Could you check a few things on this drawing? It's one solid part, dimensions in mm from its lowest x, y, z. Give positions to 0.01 mm unless a question says otherwise; leave off trailing zeros. Loops run counter-clockwise (first coordinate to the right, second up) from the corner with the lowest first, then second, coordinate; pieces in that order, holes last. Notation, with made-up numbers: M -20,35 L 5,35 A17 cw 5,43 Z; hole C -23,78.5 d5. An arc over 180 degrees is marked long. Answer in a Markdown table with one row per item. Add a question column.
1. I need wall thicknesses on line 1 along Z through (x, y) = (30, 6); line 2 along X through (y, z) = (14.25, 131); line 3 along Z through (x, y) = (31, 2.5). Which ranges of each line are inside material? Lowest first, please. Write a range as from..to.
2. If we section it at C-C on z = 130: List the corners of the cut face in (x, y) for me.
3. If we section it at B-B on y = 18.5: List the corners of the cut face in (x, z) for me, then the cut area to 3 significant figures.
4. I'm going to push a flat-ended pin straight in: pin 1 Ø12 at (x, z) = (45, 85.5) entering from -Y. Where does the tip first touch, or does it pass through?
5. If we section it at A-A on x = 30: List the corners of the cut face in (y, z) for me, then the cut area to 3 significant figures.
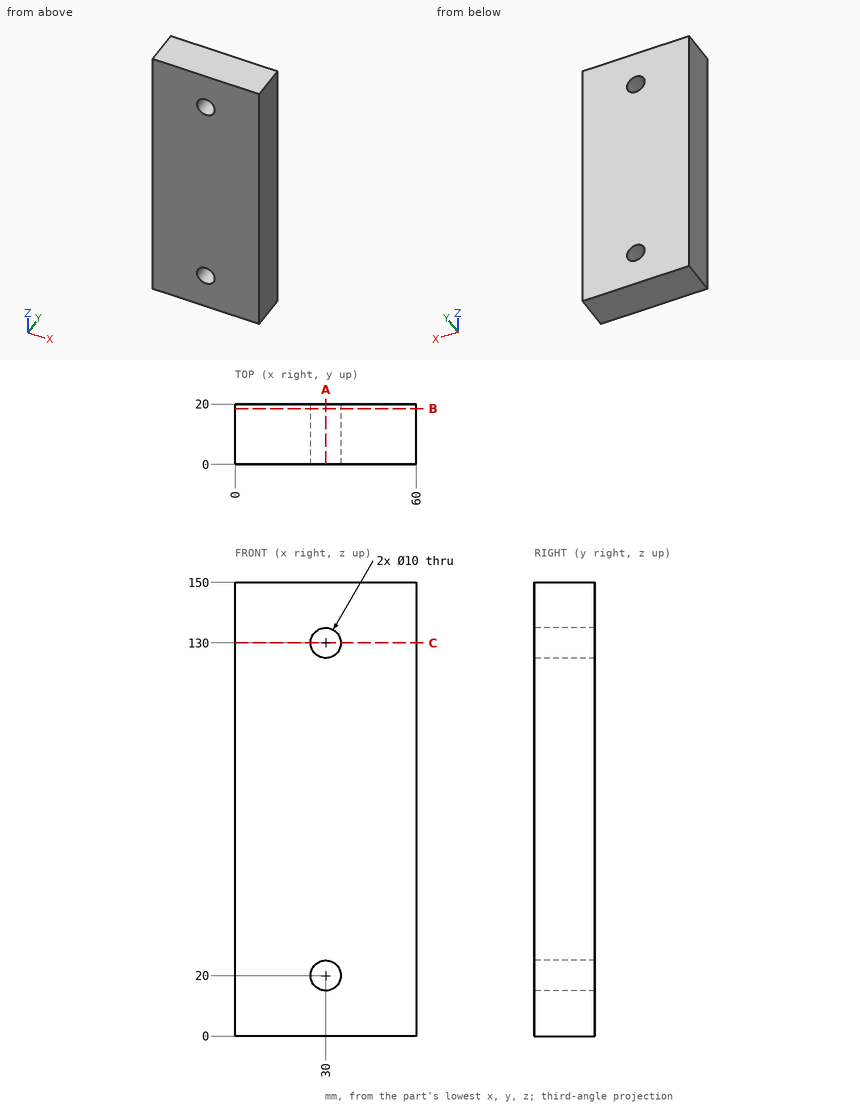
Results:
| question | item | result |
|---|---|---|
| 1 | line 1 | 0..15, 25..125, 135..150 |
| 1 | line 2 | 0..25.1, 34.9..60 |
| 1 | line 3 | 0..15.1, 24.9..125.1, 134.9..150 |
| 2 | outline | M 0,0 L 25,0 L 25,20 L 0,20 Z; M 35,0 L 60,0 L 60,20 L 35,20 Z |
| 3 | outline | M 0,0 L 60,0 L 60,150 L 0,150 Z; hole C 30,20 d10; hole C 30,130 d10 |
| 3 | area | 8,840 mm2 |
| 4 | pin 1 | y = 0 |
| 5 | outline | M 0,0 L 20,0 L 20,15 L 0,15 Z; M 0,25 L 20,25 L 20,125 L 0,125 Z; M 0,135 L 20,135 L 20,150 L 0,150 Z |
| 5 | area | 2,600 mm2 |
